from build123d import *

# Parameters (mm, degrees)
SKETCH_1_W          = 88.5
SKETCH_1_H          = 37.6
SKETCH_1_R          = 2.025
EXTRUDE_1_DEPTH     = 10
CUT_EXTRUDE_1_DEPTH = 11
CUT_EXTRUDE_2_DEPTH = 11
SKETCH_4_W          = 30
SKETCH_4_H          = 29.6
CUT_EXTRUDE_3_DEPTH = 11
SKETCH_5_W          = 30
SKETCH_5_H          = 3
EXTRUDE_2_DEPTH     = 10
FILLET_1_R          = 2
CHAMFER_1_SIZE      = 3


with BuildPart() as part:
    # 草图1 → 凸台-拉伸1 (new body)
    with BuildSketch(Plane(origin=(0, 0, 0), x_dir=(1, 0, 0), z_dir=(0, 1, 0))):
        with Locations((34.25, 0)):
            Rectangle(SKETCH_1_W, SKETCH_1_H)
        with Locations((-5, 14)):
            Circle(SKETCH_1_R, mode=Mode.SUBTRACT)
        with Locations((5, 14)):
            Circle(SKETCH_1_R, mode=Mode.SUBTRACT)
        with Locations((5, -14)):
            Circle(SKETCH_1_R, mode=Mode.SUBTRACT)
        with Locations((-5, -14)):
            Circle(SKETCH_1_R, mode=Mode.SUBTRACT)
        with Locations((45.5, 14)):
            Circle(SKETCH_1_R, mode=Mode.SUBTRACT)
        with Locations((59.5, 14)):
            Circle(SKETCH_1_R, mode=Mode.SUBTRACT)
        with Locations((73.5, 14)):
            Circle(SKETCH_1_R, mode=Mode.SUBTRACT)
        with Locations((73.5, -14)):
            Circle(SKETCH_1_R, mode=Mode.SUBTRACT)
        with Locations((59.5, -14)):
            Circle(SKETCH_1_R, mode=Mode.SUBTRACT)
        with Locations((45.5, -14)):
            Circle(SKETCH_1_R, mode=Mode.SUBTRACT)
    extrude(amount=EXTRUDE_1_DEPTH)

    # 草图2 → 切除-拉伸1 (cut, through all)
    with BuildSketch(Plane(origin=(0, 10, 0), x_dir=(1, 0, 0), z_dir=(0, 1, 0))):
        with BuildLine():
            Line((-7.5, -9.5), (-7.5, 9.5))
            ThreePointArc((-7.5, 9.5), (-7.207106781, 10.207106781), (-6.5, 10.5))
            Line((-6.5, 10.5), (-5, 10.5))
            ThreePointArc((-5, 10.5), (-2.525126266, 11.525126266), (-1.5, 14))
            Line((-1.5, 14), (-1.5, 15.3))
            ThreePointArc((-1.5, 15.3), (-1.207106781, 16.007106781), (-0.5, 16.3))
            Line((-0.5, 16.3), (0.5, 16.3))
            ThreePointArc((0.5, 16.3), (1.207106781, 16.007106781), (1.5, 15.3))
            Line((1.5, 15.3), (1.5, 14))
            ThreePointArc((1.5, 14), (2.525126266, 11.525126266), (5, 10.5))
            Line((5, 10.5), (6.5, 10.5))
            ThreePointArc((6.5, 10.5), (7.207106781, 10.207106781), (7.5, 9.5))
            Line((7.5, 9.5), (7.5, -9.5))
            ThreePointArc((7.5, -9.5), (7.207106781, -10.207106781), (6.5, -10.5))
            Line((6.5, -10.5), (5, -10.5))
            ThreePointArc((5, -10.5), (2.525126266, -11.525126266), (1.5, -14))
            Line((1.5, -14), (1.5, -15.3))
            ThreePointArc((1.5, -15.3), (1.207106781, -16.007106781), (0.5, -16.3))
            Line((0.5, -16.3), (-0.5, -16.3))
            ThreePointArc((-0.5, -16.3), (-1.207106781, -16.007106781), (-1.5, -15.3))
            Line((-1.5, -15.3), (-1.5, -14))
            ThreePointArc((-1.5, -14), (-2.525126266, -11.525126266), (-5, -10.5))
            Line((-5, -10.5), (-6.5, -10.5))
            ThreePointArc((-6.5, -10.5), (-7.207106781, -10.207106781), (-7.5, -9.5))
        make_face()
    extrude(amount=-CUT_EXTRUDE_1_DEPTH, mode=Mode.SUBTRACT)

    # 草图3 → 切除-拉伸2 (cut, through all)
    with BuildSketch(Plane.XZ):
        with BuildLine():
            Line((43.5, -9.5), (43.5, 9.5))
            ThreePointArc((43.5, 9.5), (43.792893219, 10.207106781), (44.5, 10.5))
            Line((44.5, 10.5), (45.5, 10.5))
            ThreePointArc((45.5, 10.5), (47.974873734, 11.525126266), (49, 14))
            Line((49, 14), (49, 15.3))
            ThreePointArc((49, 15.3), (49.292893219, 16.007106781), (50, 16.3))
            Line((50, 16.3), (55, 16.3))
            ThreePointArc((55, 16.3), (55.707106781, 16.007106781), (56, 15.3))
            Line((56, 15.3), (56, 14))
            ThreePointArc((56, 14), (59.5, 10.5), (63, 14))
            Line((63, 14), (63, 15.3))
            ThreePointArc((63, 15.3), (63.292893219, 16.007106781), (64, 16.3))
            Line((64, 16.3), (69, 16.3))
            ThreePointArc((69, 16.3), (69.707106781, 16.007106781), (70, 15.3))
            Line((70, 15.3), (70, 14))
            ThreePointArc((70, 14), (71.025126266, 11.525126266), (73.5, 10.5))
            Line((73.5, 10.5), (74.5, 10.5))
            ThreePointArc((74.5, 10.5), (75.207106781, 10.207106781), (75.5, 9.5))
            Line((75.5, 9.5), (75.5, -9.5))
            ThreePointArc((75.5, -9.5), (75.207106781, -10.207106781), (74.5, -10.5))
            Line((74.5, -10.5), (73.5, -10.5))
            ThreePointArc((73.5, -10.5), (71.025126266, -11.525126266), (70, -14))
            Line((70, -14), (70, -15.3))
            ThreePointArc((70, -15.3), (69.707106781, -16.007106781), (69, -16.3))
            Line((69, -16.3), (64, -16.3))
            ThreePointArc((64, -16.3), (63.292893219, -16.007106781), (63, -15.3))
            Line((63, -15.3), (63, -14))
            ThreePointArc((63, -14), (59.5, -10.5), (56, -14))
            Line((56, -14), (56, -15.3))
            ThreePointArc((56, -15.3), (55.707106781, -16.007106781), (55, -16.3))
            Line((55, -16.3), (50, -16.3))
            ThreePointArc((50, -16.3), (49.292893219, -16.007106781), (49, -15.3))
            Line((49, -15.3), (49, -14))
            ThreePointArc((49, -14), (47.974873734, -11.525126266), (45.5, -10.5))
            Line((45.5, -10.5), (44.5, -10.5))
            ThreePointArc((44.5, -10.5), (43.792893219, -10.207106781), (43.5, -9.5))
        make_face()
    extrude(amount=-CUT_EXTRUDE_2_DEPTH, mode=Mode.SUBTRACT)

    # 草图4 → 切除-拉伸3 (cut, through all)
    with BuildSketch(Plane.XZ):
        with Locations((25.5, 0)):
            Rectangle(SKETCH_4_W, SKETCH_4_H)
    extrude(amount=-CUT_EXTRUDE_3_DEPTH, mode=Mode.SUBTRACT)

    # 草图5 → 凸台-拉伸2 (add)
    with BuildSketch(Plane.XZ):
        with Locations((25.5, 0)):
            Rectangle(SKETCH_5_W, SKETCH_5_H)
    extrude(amount=-EXTRUDE_2_DEPTH)

    # 圆角1
    fillet_1_edges = [part.edges().sort_by_distance(p)[0] for p in [
        (40.5, 5, 14.8),
        (40.5, 5, -14.8),
        (10.5, 5, -14.8),
        (10.5, 5, 14.8),
        (40.5, 5, -1.5),
        (40.5, 5, 1.5),
        (10.5, 5, 1.5),
        (10.5, 5, -1.5),
    ]]
    fillet(fillet_1_edges, radius=FILLET_1_R)

    # 倒角1
    chamfer_1_edges = [part.edges().sort_by_distance(p)[0] for p in [
        (-10, 5, -18.8),
        (78.5, 5, -18.8),
        (78.5, 5, 18.8),
        (-10, 5, 18.8),
    ]]
    chamfer(chamfer_1_edges, length=CHAMFER_1_SIZE)


solid = part.part
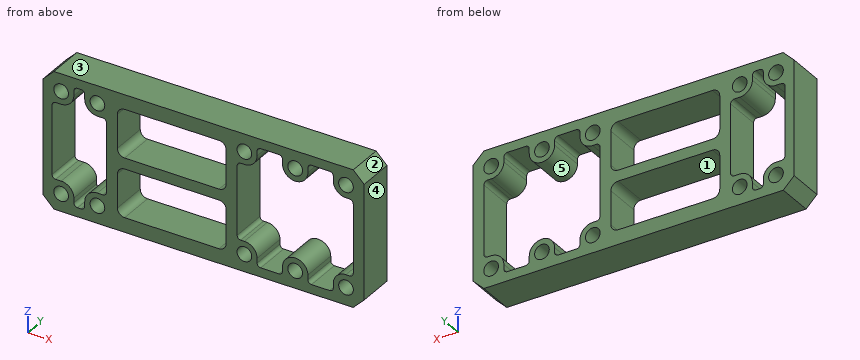
Geometry: final body of the model. Coordinates: model frame, mm. Face numbers are marked on the shaded views. A direction names the side the tool comes from. Coordinates: 2 decimals unless noted, no trailing zeros. Order: outer loops, then holes, each group sorted by start corner. A loop starts at its lowest first (then second) coordinate and runs counter-clockwise, first axis right, second up. Notation, with made-up numbers: M 88,38.5 L 123,38.5 A18 cw 123,42.5 Z; hole C -7.5,-20.5 d5. An arc over 180 degrees is marked long. One line per question, with ' | ' between items. Start each with the question number.
Item 1: Draft query along X for the marked faces 3, 4 and 5. Return one class per face: released by +X, released by -X, zero draft, split by the parting line, or undercut.
Item 2: Pin query (flat end, axial travel): pin 1 Ø3 at (x, z) = (-5, 14) entering from -Y. Return the tip coordinate at first contact, or that it passes through.
Item 3: Cut plane A-A, the plane z = 4.5. Return the cut outline in (x, y), then the cut area to 3 significant figures.
Item 4: Cut plane B-B, the plane x = 59.5. Return the cut outline in (y, z) (3 decimals).
Item 5: Ray query, probe 1 along Z at (x, y) = (5, 5) (3 decimals); probe 2 along Z at (x, y) = (51, 1.5); probe 3 along X at (y, z) = (1.5, -11). Return the intervals inside material, ascending. Write a range as [from, to].
Item 6: Set-up query: the marked faces 1 and 2. Return all of +Z, -Z, +X, -X, +Y, -Y with unobstructed straight access to the full face (end or side cutting, diameter ignored); none if empty.
Item 7: Cut plane C-C, the plane y = 2. Count the separate pieces of the cut face and the enclosed holes in it, then the cut area to 3 significant figures.
A:
1) face 3: zero draft | face 4: released by +X | face 5: undercut
2) pin 1: passes through
3) outline: M -10,0 L -7.5,0 L -7.5,10 L -10,10 Z; M 7.5,0 L 10.5,0 L 10.5,10 L 7.5,10 Z; M 40.5,0 L 43.5,0 L 43.5,10 L 40.5,10 Z; M 75.5,0 L 78.5,0 L 78.5,10 L 75.5,10 Z | area: 115 mm2
4) outline: M 0,-18.8 L 10,-18.8 L 10,-16.025 L 0,-16.025 Z; M 0,-11.975 L 10,-11.975 L 10,-10.5 L 0,-10.5 Z; M 0,10.5 L 10,10.5 L 10,11.975 L 0,11.975 Z; M 0,16.025 L 10,16.025 L 10,18.8 L 0,18.8 Z
5) probe 1: z = [-18.8, -16.025], [-11.975, -10.5], [10.5, 11.975], [16.025, 18.8] | probe 2: z = [-18.8, -16.3], [16.3, 18.8] | probe 3: x = [-10, -3.2], [3.2, 10.5], [40.5, 47.3], [57.7, 61.3], [71.7, 78.5]
6) face 1: +Y, -Y | face 2: +Z, +X, +Y, -Y
7) separate pieces: 1 | enclosed holes: 14 | area: 1,180 mm2
